from build123d import *

# Parameters (mm, degrees)
SKETCH1_W                = 60
SKETCH1_H                = 60
BOSS_EXTRUDE1_DEPTH      = 5
SKETCH2_R                = 2
CUT_EXTRUDE2_DEPTH       = 43.720018727
SKETCH8_R                = 4.5
CUT_EXTRUDE4_DEPTH       = 43.720018727
SKETCH31_R               = 1.5
CUT_EXTRUDE20_DEPTH      = 10
SKETCH33_R               = 2.5
CUT_EXTRUDE21_DEPTH      = 3
BOSS_EXTRUDE11_START     = -5
SKETCH35_R               = 4.5
SKETCH35_R_2             = 2
BOSS_EXTRUDE11_DEPTH     = 5
SKETCH37_R               = 1.5
CUT_EXTRUDE22_DEPTH      = 5
SKETCH38_R               = 2.55
CUT_EXTRUDE23_DEPTH      = 4
SKETCH7_R                = 2
CUT_EXTRUDE24_DEPTH      = 10
BOSS_EXTRUDE12_DEPTH     = 30
SKETCH40_R               = 2
CUT_EXTRUDE25_DEPTH      = 6
MIRROR20_COPY_1_SKETCH_R = 2
MIRROR20_COPY_1_DEPTH    = 6
CUT_EXTRUDE27_DEPTH      = 10


with BuildPart() as part:
    # Sketch1 → Boss-Extrude1 (new body)
    with BuildSketch(Plane(origin=(0, 0, 0), x_dir=(1, 0, 0), z_dir=(0, 1, 0))):
        Rectangle(SKETCH1_W, SKETCH1_H)
    extrude(amount=BOSS_EXTRUDE1_DEPTH)

    # Sketch2 → Cut-Extrude2 (cut, through all)
    with BuildSketch(Plane(origin=(0, 5, 0), x_dir=(1, 0, 0), z_dir=(0, 1, 0))):
        with Locations(Location((-16.25, 0, 0), (0, 0, 270))):
            Circle(SKETCH2_R)
        with Locations(Location((16.25, 0, 0), (0, 0, 90))):
            Circle(SKETCH2_R)
        with Locations(Location((0, -16.25, 0), (0, 0, 270))):
            Circle(SKETCH2_R)
        with Locations(Location((0, 16.25, 0), (0, 0, 90))):
            Circle(SKETCH2_R)
    extrude(amount=-CUT_EXTRUDE2_DEPTH, mode=Mode.SUBTRACT)

    # Sketch8 → Cut-Extrude4 (cut, through all)
    with BuildSketch(Plane(origin=(0, 5, 0), x_dir=(1, 0, 0), z_dir=(0, 1, 0))):
        with Locations(Location((0, 0, 0), (0, 0, 270))):
            Circle(SKETCH8_R)
    extrude(amount=-CUT_EXTRUDE4_DEPTH, mode=Mode.SUBTRACT)

    # Sketch31 → Cut-Extrude20 (cut)
    with BuildSketch(Plane(origin=(0, 5, 0), x_dir=(1, 0, 0), z_dir=(0, 1, 0))):
        with Locations(Location((0, 9.5, 0), (0, 0, 270))):
            Circle(SKETCH31_R)
    cut_extrude20 = extrude(amount=-CUT_EXTRUDE20_DEPTH, mode=Mode.SUBTRACT)

    # Sketch33 → Cut-Extrude21 (cut)
    with BuildSketch(Plane.XZ):
        with Locations(Location((0, -9.5, 0), (0, 0, 270))):
            Circle(SKETCH33_R)
    cut_extrude21 = extrude(amount=-CUT_EXTRUDE21_DEPTH, mode=Mode.SUBTRACT)

    # Mirror17: Cut-Extrude20, Cut-Extrude21 across plane
    add(cut_extrude20.mirror(Plane.XY), mode=Mode.SUBTRACT)
    add(cut_extrude21.mirror(Plane.XY), mode=Mode.SUBTRACT)

    # Sketch35 → Boss-Extrude11 (add)
    with BuildSketch(Plane.XZ.offset(BOSS_EXTRUDE11_START)):
        Polygon((-3.829271912, -6.598130063), (-3.829271912, -19.146359559), (3.475800658, -19.146359559), (3.475800658, -6.598130063), (6.745409752, -3.328520969), (18.851800181, -3.328520969), (18.851800181, 3.652536285), (6.745409752, 3.652536285), (3.873455818, 6.524490219), (3.873455818, 19.323095186), (-3.240153156, 19.323095186), (-3.240153156, 7.246160695), (-6.362482561, 3.652536285), (-19.676566439, 3.652536285), (-19.676566439, -3.328520969), (-6.362482561, -3.328520969), align=None)
        with Locations(Location((0, 0, 0), (0, 0, 90))):
            Circle(SKETCH35_R, mode=Mode.SUBTRACT)
        with Locations(Location((-16.25, 0, 0), (0, 0, 90))):
            Circle(SKETCH35_R_2, mode=Mode.SUBTRACT)
        with Locations(Location((0, 16.25, 0), (0, 0, 90))):
            Circle(SKETCH35_R_2, mode=Mode.SUBTRACT)
        with Locations(Location((16.25, 0, 0), (0, 0, 270))):
            Circle(SKETCH35_R_2, mode=Mode.SUBTRACT)
        with Locations(Location((0, -16.25, 0), (0, 0, 270))):
            Circle(SKETCH35_R_2, mode=Mode.SUBTRACT)
    extrude(amount=BOSS_EXTRUDE11_DEPTH)

    # Sketch37 → Cut-Extrude22 (cut)
    with BuildSketch(Plane.XZ):
        with Locations(Location((0, 8.13, 0), (0, 0, 270))):
            Circle(SKETCH37_R)
        with Locations(Location((9.5, 0, 0), (0, 0, 270))):
            Circle(SKETCH37_R)
        with Locations(Location((-9.5, 0, 0), (0, 0, 90))):
            Circle(SKETCH37_R)
        with Locations(Location((0, -8.13, 0), (0, 0, 90))):
            Circle(SKETCH37_R)
    extrude(amount=-CUT_EXTRUDE22_DEPTH, mode=Mode.SUBTRACT)

    # Sketch38 → Cut-Extrude23 (cut)
    with BuildSketch(Plane.XZ):
        with Locations(Location((0, 8.13, 0), (0, 0, 270))):
            Circle(SKETCH38_R)
        with Locations(Location((9.5, 0, 0), (0, 0, 270))):
            Circle(SKETCH38_R)
        with Locations(Location((0, -8.13, 0), (0, 0, 270))):
            Circle(SKETCH38_R)
        with Locations(Location((-9.5, 0, 0), (0, 0, 270))):
            Circle(SKETCH38_R)
    extrude(amount=-CUT_EXTRUDE23_DEPTH, mode=Mode.SUBTRACT)

    # Sketch7 → Cut-Extrude24 (cut)
    with BuildSketch(Plane(origin=(0, 5, 0), x_dir=(1, 0, 0), z_dir=(0, 1, 0))):
        with Locations(Location((-25, 0, 0), (0, 0, 270))):
            Circle(SKETCH7_R)
        with Locations(Location((0, 25, 0), (0, 0, 270))):
            Circle(SKETCH7_R)
        with Locations(Location((25, 0, 0), (0, 0, 270))):
            Circle(SKETCH7_R)
        with Locations(Location((0, -25, 0), (0, 0, 270))):
            Circle(SKETCH7_R)
        Polygon((-30, 30), (-30, 10), (-10, 30), align=None)
        Polygon((30, 30), (30, 10), (10, 30), align=None)
        Polygon((30, -30), (10, -30), (30, -10), align=None)
        Polygon((-30, -30), (-30, -10), (-10, -30), align=None)
    extrude(amount=-CUT_EXTRUDE24_DEPTH, mode=Mode.SUBTRACT)

    # Sketch39 → Boss-Extrude12 (add)
    with BuildSketch(Plane(origin=(0, 5, 0), x_dir=(1, 0, 0), z_dir=(0, 1, 0))):
        with BuildLine():
            Line((-10, 30), (10, 30))
            Line((10, 30), (15.766907344, 24.233092656))
            Line((15.766907344, 24.233092656), (10, 18.466185313))
            ThreePointArc((10, 18.466185313), (0, 21), (-10, 18.466185313))
            Line((-10, 18.466185313), (-15.766907344, 24.233092656))
            Line((-15.766907344, 24.233092656), (-10, 30))
        make_face()
        with BuildLine():
            Line((30, 10), (30, -10))
            Line((30, -10), (24.233092656, -15.766907344))
            Line((24.233092656, -15.766907344), (18.466185313, -10))
            ThreePointArc((18.466185313, -10), (21, 0), (18.466185313, 10))
            Line((18.466185313, 10), (24.233092656, 15.766907344))
            Line((24.233092656, 15.766907344), (30, 10))
        make_face()
        with BuildLine():
            Line((10, -30), (-10, -30))
            Line((-10, -30), (-15.766907344, -24.233092656))
            Line((-15.766907344, -24.233092656), (-10, -18.466185313))
            ThreePointArc((-10, -18.466185313), (0, -21), (10, -18.466185313))
            Line((10, -18.466185313), (15.766907344, -24.233092656))
            Line((15.766907344, -24.233092656), (10, -30))
        make_face()
        with BuildLine():
            Line((-30, -10), (-30, 10))
            Line((-30, 10), (-24.233092656, 15.766907344))
            Line((-24.233092656, 15.766907344), (-18.466185313, 10))
            ThreePointArc((-18.466185313, 10), (-21, 0), (-18.466185313, -10))
            Line((-18.466185313, -10), (-24.233092656, -15.766907344))
            Line((-24.233092656, -15.766907344), (-30, -10))
        make_face()
    extrude(amount=BOSS_EXTRUDE12_DEPTH)

    # Sketch40 → Cut-Extrude25 (cut)
    with BuildSketch(Plane(origin=(0, 35, 0), x_dir=(1, 0, 0), z_dir=(0, 1, 0))):
        with Locations(Location((-25, 0, 0), (0, 0, 270))):
            Circle(SKETCH40_R)
    cut_extrude25 = extrude(amount=-CUT_EXTRUDE25_DEPTH, mode=Mode.SUBTRACT)

    # Mirror19: Cut-Extrude25 across plane
    add(cut_extrude25.mirror(Plane(origin=(0, 0, 0), x_dir=(0, 0, 1), z_dir=(1, 0, 0))), mode=Mode.SUBTRACT)

    # Mirror20: Cut-Extrude25 across plane
    add(cut_extrude25.mirror(Plane(origin=(0, 0, 0), x_dir=(0.7071067811865478, 0, 0.7071067811865472), z_dir=(0.7071067811865475, 0, -0.7071067811865477))), mode=Mode.SUBTRACT)

    # Mirror20 copy 1 sketch → Mirror20 copy 1 (cut)
    with BuildSketch(Plane(origin=(0, 35, 0), x_dir=(0, 0, -1), z_dir=(0, 1, 0))):
        with Locations(Location((-25, 0, 0), (0, 0, 270))):
            Circle(MIRROR20_COPY_1_SKETCH_R)
    extrude(amount=-MIRROR20_COPY_1_DEPTH, mode=Mode.SUBTRACT)

    # Sketch42 → Cut-Extrude27 (cut)
    with BuildSketch(Plane(origin=(0, 5, 0), x_dir=(1, 0, 0), z_dir=(0, 1, 0))):
        with BuildLine():
            Line((-22.116546328, 17.883453672), (-15.383807976, 11.15071532))
            ThreePointArc((-15.383807976, 11.15071532), (-13.430193311, 13.439862634), (-11.139640554, 15.391829272))
            Line((-11.139640554, 15.391829272), (-17.873905641, 22.126094359))
            Line((-17.873905641, 22.126094359), (-22.116546328, 17.883453672))
        make_face()
        with BuildLine():
            Line((22.126094359, 17.873905641), (17.883453672, 22.116546328))
            Line((17.883453672, 22.116546328), (11.15071532, 15.383807976))
            ThreePointArc((11.15071532, 15.383807976), (13.439862634, 13.430193311), (15.391829272, 11.139640554))
            Line((15.391829272, 11.139640554), (22.126094359, 17.873905641))
        make_face()
        with BuildLine():
            Line((17.873905641, -22.126094359), (22.116546328, -17.883453672))
            Line((22.116546328, -17.883453672), (15.383807976, -11.15071532))
            ThreePointArc((15.383807976, -11.15071532), (13.430193311, -13.439862634), (11.139640554, -15.391829272))
            Line((11.139640554, -15.391829272), (17.873905641, -22.126094359))
        make_face()
        with BuildLine():
            Line((-22.126094359, -17.873905641), (-17.883453672, -22.116546328))
            Line((-17.883453672, -22.116546328), (-11.15071532, -15.383807976))
            ThreePointArc((-11.15071532, -15.383807976), (-13.439862634, -13.430193311), (-15.391829272, -11.139640554))
            Line((-15.391829272, -11.139640554), (-22.126094359, -17.873905641))
        make_face()
    extrude(amount=-CUT_EXTRUDE27_DEPTH, mode=Mode.SUBTRACT)


solid = part.part
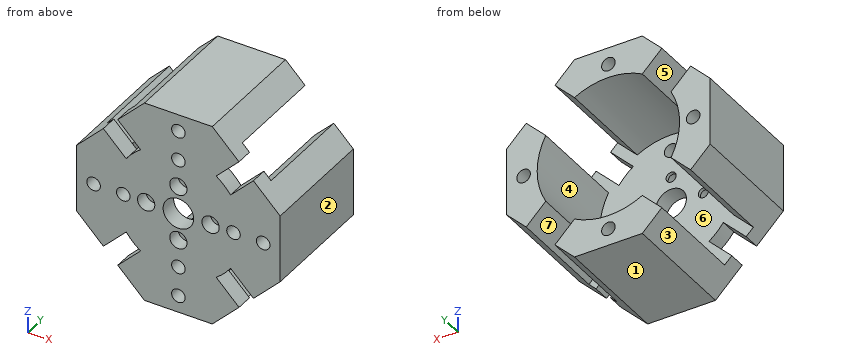
Can you work these out from the model? Positions are in its coordinate system, mm. Face numbers are marked on the shaded views. A direction names the side the tool comes from. Give positions to 0.01 mm unless a question says otherwise; leave off trailing zeros. Loops run counter-clockwise (first coordinate to the right, second up) from the corner with the lowest first, then second, coordinate; pieces in that order, holes last. Notation, with made-up numbers: M 61.5,-18.5 L 72.5,-18.5 A23 ccw 72.5,15.5 Z; hole C 60.5,55.25 d9. An arc over 180 degrees is marked long. One line per item, written item: value. Start each with the question number.
1) If we section it at D-D, the plane z = 0: Give the number of separate pieces and of enclosed holes in the cut face, and give its area (3 significant figures).
2) If I drill on line 1 (X direction, y = 16.5, z = 8.5); line 2 (Y direction, x = 14.5, z = -20); line 3 (Z direction, x = 3.5, y = 30.5), over which ranges is the centre line in solid material (lowest first)? Write a range as [from, to].
3) On a 3-axis mill with a long thin cutter (end or side, diameter ignored), from which of +Z, -Z, +X, -X, +Y, -Y can I reach the whole of each face in a straight line? I mean the marked faces 5, 6 and 7. Say none if no direction works.
4) If we section it at C-C, the plane x = -25: Write out the boundary of the cut face in (y, z), and give its area (3 significant figures).
5) Thinking about a two-plate mould opening in X: for the marked faces 1, 2, 3 and 4, which applies, +X half, -X half, draft (parallel to the pull), parting line (faces both ways), or undercut?
6) If we section it at B-B, the plane z = 25: Write out the boundary of the cut face in (x, y).
7) If we section it at A-A, the plane y = 27: Write out the boundary of the cut face in (x, z).
8) I'm going to push flat-ended pins straight in: pin 1 (12 mm diameter, centred on x = 13, y = 25.5, fed in from +Z); pin 2 (2.5 mm diameter, centred on x = 0, z = -8.13, fed in from -Y) (3 decimals); pin 3 (8 mm diameter, centred on x = 9.5, z = 0, fed in from +Y); pin 4 (3 mm diameter, centred on x = 25, z = 0, fed in from +Y). Where does each tip first touch, or does it pass through?
Completed:
1. separate pieces: 6
1. enclosed holes: 0
1. area: 620 mm^2
2. line 1: x = [-30, -19.2], [19.2, 30]
2. line 2: y = [0, 5]
2. line 3: z = [-30, -20.71], [20.71, 30]
3. face 5: -X, +Y
3. face 6: +Y
3. face 7: -Z, +Y
4. outline: M 0,-15 L 35,-15 L 35,-2 L 29,-2 L 29,2 L 35,2 L 35,15 L 0,15 L 0,2 L 5,2 L 5,-2 L 0,-2 Z
4. area: 1,010 mm^2
5. face 1: draft
5. face 2: +X half
5. face 3: -X half
5. face 4: undercut
6. outline: M -15,0 L -2,0 L -2,5 L 2,5 L 2,0 L 15,0 L 15,35 L 2,35 L 2,29 L -2,29 L -2,35 L -15,35 Z
7. outline: M -30,-10 L -24.23,-15.77 L -18.47,-10 A21 cw -18.47,10 L -24.23,15.77 L -30,10 Z; M -15.77,-24.23 L -10,-30 L 10,-30 L 15.77,-24.23 L 10,-18.47 A21 cw -10,-18.47 Z; M -15.77,24.23 L -10,18.47 A21 cw 10,18.47 L 15.77,24.23 L 10,30 L -10,30 Z; M 18.47,-10 L 24.23,-15.77 L 30,-10 L 30,10 L 24.23,15.77 L 18.47,10 A21 cw Z
8. pin 1: stops at z = 30
8. pin 2: passes through
8. pin 3: stops at y = 5
8. pin 4: stops at y = 29
